```python
from build123d import *

# Parameters (mm, degrees)
SKETCH1_R                             = 11.1125
SKETCH1_R_2                           = 6.35
BOSS_EXTRUDE1_DEPTH                   = 12.7
SKETCH4_R                             = 3.1623
BOSS_EXTRUDE2_DEPTH                   = 6.35
SKETCH5_W                             = 12.7
SKETCH5_H                             = 6.35
CUT_EXTRUDE1_DEPTH                    = 30.185832393
CIRPATTERN1_COUNT                     = 3
FILLET2_R                             = 3.175
BOSS_EXTRUDE3_START                   = -12.7
BOSS_EXTRUDE3_DEPTH                   = 12.7
CUT_EXTRUDE2_REACH                    = 43.809
CUT_EXTRUDE3_DEPTH                    = 42.808737587
CUT_EXTRUDE3_DEPTH_BACK               = 42.808737587
TAPPED_HOLE_FOR_10_32_HELICOIL1_D     = 5.1054
TAPPED_HOLE_FOR_10_32_HELICOIL1_DEPTH = 11.9888
TAPPED_HOLE_FOR_10_32_HELICOIL1_TIP   = 1.533816902


# Read off the part's stored shape, not the designer's step: Boss-Extrude3
with BuildPart() as part:
    # Sketch1 → Boss-Extrude1 (new body)
    with BuildSketch(Plane(origin=(0, 0, 0), x_dir=(1, 0, 0), z_dir=(0, 1, 0))):
        with Locations(Location((0, 0, 0), (0, 0, 270))):
            Circle(SKETCH1_R)
        with Locations(Location((0, 0, 0), (0, 0, 270))):
            Circle(SKETCH1_R_2, mode=Mode.SUBTRACT)
    extrude(amount=BOSS_EXTRUDE1_DEPTH)

    # Sketch4 → Boss-Extrude2 (add, symmetric)
    with BuildSketch(Plane.XY):
        Polygon((11.1125, 12.7), (23.8125, 9.297045256), (23.8125, 3.402954744), (23.8125, 0), (11.1125, 0), (8.73125, 0), (8.73125, 12.7), align=None)
        with Locations((17.4625, 6.35)):
            Circle(SKETCH4_R, mode=Mode.SUBTRACT)
    boss_extrude2 = extrude(amount=BOSS_EXTRUDE2_DEPTH, both=True)

    # Sketch5 → Cut-Extrude1 (cut, through all)
    with BuildSketch(Plane(origin=(0, 12.7, 0), x_dir=(1, 0, 0), z_dir=(0, 1, 0))):
        with Locations((17.4625, 0)):
            Rectangle(SKETCH5_W, SKETCH5_H)
    cut_extrude1 = extrude(amount=-CUT_EXTRUDE1_DEPTH, mode=Mode.SUBTRACT)

    # CirPattern1: Boss-Extrude2, Cut-Extrude1 ×3 about axis
    cirpattern1_axis = Axis((0, 0, 0), (0, 1, 0))
    add([boss_extrude2.rotate(cirpattern1_axis, i * 360 / CIRPATTERN1_COUNT) for i in range(1, CIRPATTERN1_COUNT)])
    add([cut_extrude1.rotate(cirpattern1_axis, i * 360 / CIRPATTERN1_COUNT) for i in range(1, CIRPATTERN1_COUNT)], mode=Mode.SUBTRACT)

    # Fillet2
    fillet2_edges = [part.edges().sort_by_distance(p)[0] for p in [
        (9.119493201, 6.35, -6.35),
        (9.119493201, 6.35, 6.35),
        (-16.030695986, 9.297045256, -18.240979928),
        (-16.030695986, 0, -18.240979928),
        (-7.781804014, 9.297045256, 23.003479928),
        (-7.781804014, 0, 23.003479928),
        (23.8125, 9.297045256, 4.7625),
        (23.8125, 0, 4.7625),
        (23.8125, 9.297045256, -4.7625),
        (23.8125, 0, -4.7625),
        (0.939514713, 6.35, 11.072712782),
        (-16.030695986, 9.297045256, 18.240979928),
        (-16.030695986, 0, 18.240979928),
        (0.939514713, 6.35, -11.072712782),
        (-7.781804014, 9.297045256, -23.003479928),
        (-7.781804014, 0, -23.003479928),
    ]]
    fillet(fillet2_edges, radius=FILLET2_R)

    # Boss-Extrude3 outline → Boss-Extrude3 (add)
    with BuildSketch(Plane(origin=(0, 12.7, 0), x_dir=(1, 0, 0), z_dir=(0, 1, 0)).offset(BOSS_EXTRUDE3_START)):
        with BuildLine():
            ThreePointArc((-10.059007915, -4.722712782), (-10.845929691, -2.419393601), (-11.1125, 0))
            Line((-11.1125, 0), (-11.1125, -4.722712782))
            ThreePointArc((-11.1125, -4.722712782), (-11.337716442, -6.459773203), (-11.99847248, -8.081963948))
            Line((-11.99847248, -8.081963948), (-11.055511314, -6.4487073))
            Line((-11.055511314, -6.4487073), (-10.059007915, -4.722712782))
        make_face()
        with BuildLine():
            Line((-11.055511314, 6.4487073), (-11.99847248, 8.081963948))
            ThreePointArc((-11.99847248, 8.081963948), (-11.337716442, 6.459773203), (-11.1125, 4.722712782))
            Line((-11.1125, 4.722712782), (-11.1125, 0))
            ThreePointArc((-11.1125, 0), (-10.845929691, 2.419393601), (-10.059007915, 4.722712782))
            Line((-10.059007915, 4.722712782), (-11.055511314, 6.4487073))
        make_face()
    extrude(amount=BOSS_EXTRUDE3_DEPTH)

    # Sketch9 → Cut-Extrude2 (cut, up to next)
    with BuildSketch(Plane(origin=(-5.499261314, 0, -3.175), x_dir=(-0.500000000000004, 0, 0.8660254037844364), z_dir=(-0.8660254037844365, 0, -0.500000000000004)), mode=Mode.PRIVATE) as cut_extrude2_sk1:
        Polygon((11.1125, 12.7), (12.998422331, 12.194668634), (12.998422331, 12.7), align=None)
    cut_extrude2_tool1 = extrude(cut_extrude2_sk1.sketch, amount=CUT_EXTRUDE2_REACH, mode=Mode.PRIVATE) & part.part
    add(cut_extrude2_tool1.solids().sort_by_distance((-11.684152, 12.531556, 7.537545))[0], mode=Mode.SUBTRACT)

    # Sketch10 → Cut-Extrude3 (cut, two sides: drawn at the far end of the back side and taken through both)
    with BuildSketch(Plane(origin=(-5.499261314, 0, 3.175), x_dir=(0.49999999999999195, 0, 0.8660254037844434), z_dir=(-0.8660254037844434, 0, 0.49999999999999195)).offset(-CUT_EXTRUDE3_DEPTH_BACK)):
        Polygon((-12.998422331, 117.204706423), (-12.998422331, 12.7), (-12.998422331, 12.194668634), (-11.1125, 12.7), (89.831294903, 39.747808325), (215.584349787, 206.694218426), (112.754632553, 284.151116524), align=None)
    extrude(amount=CUT_EXTRUDE3_DEPTH + CUT_EXTRUDE3_DEPTH_BACK, mode=Mode.SUBTRACT)

    # Tapped Hole for #10-32 Helicoil1
    with Locations(Plane.ZY.offset(11.1125)):
        with Locations((0, 6.35)):
            Hole(TAPPED_HOLE_FOR_10_32_HELICOIL1_D / 2, depth=TAPPED_HOLE_FOR_10_32_HELICOIL1_DEPTH)
            with Locations((0, 0, -(TAPPED_HOLE_FOR_10_32_HELICOIL1_DEPTH + TAPPED_HOLE_FOR_10_32_HELICOIL1_TIP / 2))):  # 118° drill point
                Cone(0, TAPPED_HOLE_FOR_10_32_HELICOIL1_D / 2, TAPPED_HOLE_FOR_10_32_HELICOIL1_TIP, mode=Mode.SUBTRACT)


solid = part.part
```
Verification items for the finished model (mm, model axes). A direction names the side the tool comes from. Coordinates: 2 decimals unless noted, no trailing zeros. Order: outer loops, then holes, each group sorted by start corner. A loop starts at its lowest first (then second) coordinate and runs counter-clockwise, first axis right, second up. Notation, with made-up numbers: (-21, 9.25) - (-12, 9.25) arc R33 ccw to (-12, 42.25) - close; hole circle Ø11 at (13, -8.75). An arc over 180 degrees is marked (long way). Return JSON: item names as keys, results as strings.
(1) Thickness scan on line 1 along Y through (x, z) = (-9, 0); line 2 along X through (y, z) = (6.35, 4.5); line 3 along X through (y, z) = (6.35, 4.3). Record the ranges inside material, lowest first.
Filled sheet:
{"line 1": "y = 0 to 3.8, 8.9 to 12.7", "line 2": "x = -11.11 to -4.48, 4.48 to 14.3, 20.62 to 23.81", "line 3": "x = -11.11 to -4.67, 4.67 to 14.3, 20.62 to 23.81"}
(2) Section check A-A, the plane z = 0. Record the cut outline in (x, y).
Filled sheet:
{"outline": "(-11.11, 0) - (-6.35, 0) - (-6.35, 3.8) - (-11.11, 3.8) - close; (-11.11, 8.9) - (-6.35, 8.9) - (-6.35, 12.7) - (-11.11, 12.7) - close; (6.35, 0) - (11.11, 0) - (11.11, 12.7) - (6.35, 12.7) - close"}
(3) Section check C-C, the plane z = -5.5. Give the number of separate pieces and of enclosed holes in the cut face, and give its area (3 significant figures).
Filled sheet:
{"separate pieces": "2", "enclosed holes": "1", "area": "307 mm^2"}
(4) Mould release check, pull along Z, two halves, no side actions. Record for faces 6 (the flat face through (-1.7, 0, -6.3)), 7 (the cylindrical face through (-7.426, 8.817, 22.431)), 8 (the cylindrical face through (-3.42, 8.49, 15.5)): pulls with the +Z half, pulls with the -Z half, needs draft (parallel to the pull), parting line crosses it, or undercut.
Filled sheet:
{"face 6": "needs draft", "face 7": "pulls with the +Z half", "face 8": "undercut"}
(5) Go/stop test with flat-tipped pins: pin 1 (6.5 mm diameter, centred on x = 19, y = 9.5, fed in from -Z); pin 2 (5.5 mm diameter, centred on x = 17.46, y = 6.35, fed in from -Z); pin 3 (3 mm diameter, centred on y = 5, z = -1, fed in from +X); pin 4 (14.5 mm diameter, centred on x = 0, z = 0, fed in from +Y). Record where each tip stops, or that it passes through.
Filled sheet:
{"pin 1": "stops at z = -6.35", "pin 2": "passes through", "pin 3": "stops at x = 11.11", "pin 4": "stops at y = 12.7"}
(6) Access from +Z, -Z, +X, -X, +Y, -Y to the whole of each face (thin tool, end or side, straight path). Record for faces 1 (the flat face through (14, 5, -6.35)), 2 (the flat face through (14, 5, 6.35)), 3 (the flat face through (15, 4, -3.175)), 4 (the flat face through (-15.34, 3.47, 13.87)), 5 (the cylindrical face through (-8.43, 6.46, 2.55)).
Filled sheet:
{"face 1": "-Z, +X, +Y, -Y", "face 2": "+Z, +X, +Y, -Y", "face 3": "+X, +Y, -Y", "face 4": "-X, +Y, -Y", "face 5": "-X"}
(7) Section check B-B, the plane x = 1. Record the cut outline in (y, z), and give its area (3 significant figures).
Filled sheet:
{"outline": "(0, -11.46) - (12.7, -11.46) - (12.7, -6.27) - (0, -6.27) - close; (0, 6.27) - (12.7, 6.27) - (12.7, 11.46) - (0, 11.46) - close", "area": "132 mm^2"}
